Geometry check sheet. Reference: the model listing, model coordinates, mm. A direction names the side the tool comes from. Give positions to 0.01 mm unless a question says otherwise; leave off trailing zeros. Order: outer loops, then holes, each group sorted by start corner. A loop starts at its lowest first (then second) coordinate and runs counter-clockwise, first axis right, second up. Notation, with made-up numbers: M -33,-38 L -9,-38 A16 cw -9,-8 Z; hole C -24,69.25 d8. An arc over 180 degrees is marked long. Answer as CSV lines item,"result".
from build123d import *

# Parameters (mm, degrees)
SKETCH1_R           = 12.5
BOSS_EXTRUDE1_DEPTH = 143.4
SKETCH4_W           = 8
SKETCH4_H           = 8
CUT_EXTRUDE1_DEPTH  = 35.4
SKETCH11_R          = 15.5
BOSS_EXTRUDE4_DEPTH = 2
SKETCH12_R          = 12.5
SKETCH12_R_2        = 11.75
CUT_EXTRUDE2_DEPTH  = 1.2
SKETCH13_W          = 8
SKETCH13_H          = 7
CUT_EXTRUDE3_DEPTH  = 47
SKETCH16_R          = 12.5
SKETCH16_R_2        = 11.75
CUT_EXTRUDE5_DEPTH  = 1.2


with BuildPart() as part:
    # Sketch1 → Boss-Extrude1 (new body)
    with BuildSketch(Plane.XY):
        Circle(SKETCH1_R)
    extrude(amount=BOSS_EXTRUDE1_DEPTH)

    # Sketch4 → Cut-Extrude1 (cut)
    with BuildSketch(Plane(origin=(0, 0, 0), x_dir=(-1, 0, 0), z_dir=(0, 0, -1))):
        with Locations((0, 12.5)):
            Rectangle(SKETCH4_W, SKETCH4_H)
    extrude(amount=-CUT_EXTRUDE1_DEPTH, mode=Mode.SUBTRACT)

    # Sketch11 → Boss-Extrude4 (add)
    with BuildSketch(Plane(origin=(0, 0, 37.4), x_dir=(-1, 0, 0), z_dir=(0, 0, -1))):
        Circle(SKETCH11_R)
    extrude(amount=-BOSS_EXTRUDE4_DEPTH)

    # Sketch12 → Cut-Extrude2 (cut)
    with BuildSketch(Plane.XY.offset(60)):
        Circle(SKETCH12_R)
        Circle(SKETCH12_R_2, mode=Mode.SUBTRACT)
    extrude(amount=CUT_EXTRUDE2_DEPTH, mode=Mode.SUBTRACT)

    # Sketch13 → Cut-Extrude3 (cut)
    with BuildSketch(Plane.XY.offset(143.4)):
        with Locations((0, 12.5)):
            Rectangle(SKETCH13_W, SKETCH13_H)
    extrude(amount=-CUT_EXTRUDE3_DEPTH, mode=Mode.SUBTRACT)

    # Sketch16 → Cut-Extrude5 (cut)
    with BuildSketch(Plane.XY.offset(138.4)):
        Circle(SKETCH16_R)
        Circle(SKETCH16_R_2, mode=Mode.SUBTRACT)
    extrude(amount=CUT_EXTRUDE5_DEPTH, mode=Mode.SUBTRACT)


solid = part.part
(1) Material ranges on line 1 (Z direction, x = 4.5, y = 11); line 2 (Z direction, x = -12, y = -9.5); line 3 (X direction, y = 0.5, z = 27), recorded low to high.
The answers:
line 1,"z = 0 to 60, 61.2 to 138.4, 139.6 to 143.4"
line 2,"z = 37.4 to 39.4"
line 3,"x = -12.49 to 12.49"
(2) Section check B-B on y = 0. Enter the section's corners in (x, z), then the cut area to 3 significant figures.
The answers:
outline,"M -15.5,37.4 L -12.5,37.4 L -12.5,0 L 12.5,0 L 12.5,37.4 L 15.5,37.4 L 15.5,39.4 L 12.5,39.4 L 12.5,60 L 11.75,60 L 11.75,61.2 L 12.5,61.2 L 12.5,138.4 L 11.75,138.4 L 11.75,139.6 L 12.5,139.6 L 12.5,143.4 L -12.5,143.4 L -12.5,139.6 L -11.75,139.6 L -11.75,138.4 L -12.5,138.4 L -12.5,61.2 L -11.75,61.2 L -11.75,60 L -12.5,60 L -12.5,39.4 L -15.5,39.4 Z"
area,"3,590 mm2"
(3) Gauge pin test, flat ends, axial feed: P1, Ø2, axis at x = -12, z = 100, coming from the +Y side; P2, Ø2.5, axis at y = 11, z = 111.5, coming from the -X side; P3, Ø8, axis at y = -12, z = 18, coming from the -X side. Record the tip position at first contact, or that the pin passes through.
The answers:
P1,"stops at y = 5.94"
P2,"stops at x = -7.82"
P3,"stops at x = -9.6"
(4) Draft check along X on faces 5 (the face through (5, -11, 138.4)), 6 (the face through (11.207, 3.529, 60.592)), 7 (the face through (4, 10, 120)). Enter one of: +X half, -X half, draft (parallel to the pull), parting line (faces both ways), or undercut.
The answers:
face 5,"draft"
face 6,"parting line"
face 7,"undercut"
(5) Section check A-A on x = 0. Enter the section's corners in (y, z), then the cut area to 3 significant figures.
The answers:
outline,"M -15.5,37.4 L -12.5,37.4 L -12.5,0 L 8.5,0 L 8.5,35.4 L 12.5,35.4 L 12.5,37.4 L 15.5,37.4 L 15.5,39.4 L 12.5,39.4 L 12.5,60 L 11.75,60 L 11.75,61.2 L 12.5,61.2 L 12.5,96.4 L 9,96.4 L 9,143.4 L -12.5,143.4 L -12.5,139.6 L -11.75,139.6 L -11.75,138.4 L -12.5,138.4 L -12.5,61.2 L -11.75,61.2 L -11.75,60 L -12.5,60 L -12.5,39.4 L -15.5,39.4 Z"
area,"3,290 mm2"
(6) Section check C-C on z = 132.5. Enter the section's corners in (x, y), then the cut area to 3 significant figures.
The answers:
outline,"M -4,9 L -4,11.84 A12.5 ccw long 4,11.84 L 4,9 Z"
area,"465 mm2"
(7) Tool access check on faces 1 (the face through (-4, 10, 17)), 2 (the face through (5.77, -11.09, 99.26)), 3 (the face through (-0.46, -11.74, 138.99)), 4 (the face through (-4, 10, 120)). Record the directions out of +Z, -Z, +X, -X, +Y, -Y that give a thin tool (end or side, any length) a straight path to the whole face; none if there is none.
The answers:
face 1,"-Z, +Y"
face 2,"+Z"
face 3,"none"
face 4,"+Z, +Y"
